Read the model definition and answer for the solid it produces. Units are mm, in the model's axes. A direction names the side the tool comes from. Coordinates: 2 decimals unless noted, no trailing zeros. Write each loop counter-clockwise with the first axis right and the second up, starting at its lowest first coordinate (ties: lowest second). Pieces come first, ordered by that corner, then holes. Notation, with made-up numbers: (-14, 28.5) -> (26, 28.5) arc R19 cw to (26, 51.5) -> close; hole circle Ø9 at (-4, -34.5). An arc over 180 degrees is marked (long way). Return JSON: item names as keys, results as strings.
Autodesk Inventor part; units mm, degrees
ref_plane "YZ Plane" through (0, 0, 0) normal (1, 0, 0) x (0, 1, 0)
ref_plane "XZ Plane" through (0, 0, 0) normal (0, 1, 0) x (-1, 0, 0)
ref_plane "XY Plane" through (0, 0, 0) normal (0, 0, 1) x (1, 0, 0)
sketch "Sketch1" plane through (0, 0, 0) normal (0, 0, 1) x (1, 0, 0)
  line L0 (-12.1708, 16.0073) -> (13.2292, 16.0073)
  line L1 (13.2292, 16.0073) -> (13.2292, -34.7927)
  line L2 (13.2292, -34.7927) -> (-12.1708, -34.7927)
  line L3 (-12.1708, -34.7927) -> (-12.1708, 16.0073)
  line L4 (11.9592, 14.7373) -> (-10.9008, 14.7373)
  line L5 (-10.9008, 14.7373) -> (-10.9008, -33.5227)
  line L6 (-10.9008, -33.5227) -> (11.9592, -33.5227)
  line L7 (11.9592, -33.5227) -> (11.9592, 14.7373)
  point P0 (0, 0)
  dimension "d0" = 25.4
  dimension "d1" = 50.8
  dimension "d2" = 1.27
extrude "Extrusion1" add sketch "Sketch1" along normal blind 152.4
sketch "Sketch2" plane through (-12.1708, 16.0073, 0) normal (0, 1, 0) x (1, 0, 0)
  circle A0 centre (12.7, -12.7) radius 1.7272
  line L0 (25.4, 0) -> (0, 0)
  line L1 (0, 0) -> (0, -152.4)
  point P0 (12.1708, 0)
  dimension "d5" = 3.4544
  dimension "d6" = 12.7
  dimension "d7" = 12.7
extrude "Extrusion2" cut sketch "Sketch2" against normal through all
pattern_linear "Rectangular Pattern1" count 15 spacing 25.4 along (0, 0, 1) of "Extrusion2"
sketch "Sketch3" plane through (13.2292, -34.7927, 0) normal (1, 0, 0) x (0, 0, -1)
  circle A0 centre (-38.1, 25.4) radius 9.525
  circle A1 centre (-12.7, 25.4) radius 2.5781
  circle A2 centre (-63.5, 25.4) radius 2.5781
  line L0 (0, 0) -> (0, 50.8)
  circle A3 centre (-114.3, 25.4) radius 9.525
  circle A4 centre (-88.9, 25.4) radius 2.5781
  circle A5 centre (-139.7, 25.4) radius 2.5781
  line L1 (-152.4, 0) -> (-152.4, 50.8)
  line L2 (0, 0) -> (-152.4, 0)
  line L3 (0, 50.8) -> (-152.4, 50.8) construction
  line L4 (-76.2, 50.8) -> (-76.2, 0) construction
  point P0 (0, 34.7927)
  dimension "d15" = 19.05
  dimension "d16" = 5.1562
  dimension "d17" = 5.1562
  dimension "d18" = 25.4
  dimension "d19" = 25.4
  dimension "d20" = 38.1
  dimension "d32" = 152.4
extrude "Extrusion3" cut sketch "Sketch3" against normal through all
equation "\"d3\" = d13"
equation "\"d10\" = d14"
equation "\"d13\" = 152.4"
equation "\"d14\" = d13"
properties part number "VersaFrame-Driver"
1. The part is cut by section C-C (y = -21.5). Determine the outline of the cut face in (x, z).
Taken from the geometry:
{"outline": "(-12.17, 0) -> (-10.9, 0) -> (-10.9, 152.4) -> (-12.17, 152.4) -> close; (11.96, 0) -> (13.23, 0) -> (13.23, 152.4) -> (11.96, 152.4) -> close"}
2. For a pull along Z with two mould halves and no side action, classify faces 3 (the face through (-12, -9, 152.4)), 4 (the face through (-11.527, -6.532, 105.215)), 5 (the face through (-10.901, -9, 75)) as +Z half, -Z half, draft (parallel to the pull), parting line (faces both ways), or undercut.
Taken from the geometry:
{"face 3": "+Z half", "face 4": "undercut", "face 5": "draft"}
3. A flat-ended cylindrical pin translates along its axis: pin 1 Ø3 at (x, z) = (0.53, 63.5) entering from +Y. Find the tip coordinate at first contact, or state that the pin passes through.
Taken from the geometry:
{"pin 1": "passes through"}
4. Consider L1, parallel to X at y = 15.05, z = 38.1; L2, parallel to Y at x = 9.75, z = 104; L3, parallel to X at y = 9, z = 134. Determine where each line is inside the solid, lowest interval first.
Taken from the geometry:
{"L1": "x = -12.17 to -1.2, 2.26 to 13.23", "L2": "y = -34.79 to -33.52, 14.74 to 16.01", "L3": "x = -12.17 to -10.9, 11.96 to 13.23"}
5. The part is cut by section A-A (x = -6). Determine the outline of the cut face in (y, z).
Taken from the geometry:
{"outline": "(-34.79, 0) -> (-33.52, 0) -> (-33.52, 152.4) -> (-34.79, 152.4) -> close; (14.74, 0) -> (16.01, 0) -> (16.01, 152.4) -> (14.74, 152.4) -> close"}
6. The part is cut by section D-D (z = 46). Determine the outline of the cut face in (x, y).
Taken from the geometry:
{"outline": "(-12.17, -34.79) -> (13.23, -34.79) -> (13.23, -14.71) -> (11.96, -14.71) -> (11.96, -33.52) -> (-10.9, -33.52) -> (-10.9, -14.71) -> (-12.17, -14.71) -> close; (-12.17, -4.07) -> (-10.9, -4.07) -> (-10.9, 14.74) -> (11.96, 14.74) -> (11.96, -4.07) -> (13.23, -4.07) -> (13.23, 16.01) -> (-12.17, 16.01) -> close"}
7. A tool of negligible diameter and unlimited length cuts with its end or side. For faces 1 (the face through (0, -33.523, 75)), 2 (the face through (-11.53, -10.38, 61.12)), from which of +Z, -Z, +X, -X, +Y, -Y can it reach the whole face along a straight path? Write none if from no direction.
Taken from the geometry:
{"face 1": "+Z, -Z", "face 2": "+X, -X"}
8. The part is cut by section B-B (z = 88.9). Determine the outline of the cut face in (x, y).
Taken from the geometry:
{"outline": "(-12.17, -34.79) -> (-1.2, -34.79) -> (-1.2, -33.52) -> (-10.9, -33.52) -> (-10.9, -11.97) -> (-12.17, -11.97) -> close; (-12.17, -6.81) -> (-10.9, -6.81) -> (-10.9, 14.74) -> (-1.2, 14.74) -> (-1.2, 16.01) -> (-12.17, 16.01) -> close; (2.26, -34.79) -> (13.23, -34.79) -> (13.23, -11.97) -> (11.96, -11.97) -> (11.96, -33.52) -> (2.26, -33.52) -> close; (2.26, 14.74) -> (11.96, 14.74) -> (11.96, -6.81) -> (13.23, -6.81) -> (13.23, 16.01) -> (2.26, 16.01) -> close"}
